Input: part model. Units: mm. Frame: model coordinates. A direction names the side the tool comes from. Coordinates: 2 decimals unless noted, no trailing zeros. Order: outer loops, then holes, each group sorted by start corner. A loop starts at its lowest first (then second) coordinate and runs counter-clockwise, first axis right, second up. Notation, with made-up numbers: (84.25, 65) - (123.25, 65) arc R34 cw to (123.25, 100) - close; hole circle Ø7 at (-0.5, 13). An arc over 180 degrees is marked (long way). Answer as CSV lines item,"result". Start each with the question number.
Item 1: First-contact query: pin 1 (6 mm diameter, centred on y = 2, z = 8.5, fed in from +X); pin 2 (10 mm diameter, centred on x = 57.5, y = 29.5, fed in from -Z); pin 3 (10 mm diameter, centred on x = 17, z = 5, fed in from -Y). Flat tips, straight axial feed; report the tip coordinate or a pass-through.
Item 2: Section C-C (x = 61). Output: boundary loops of the cut face in (y, z), and give its area (3 significant figures).
Item 3: Section D-D (z = 2.5). Output: boundary loops of the cut face in (x, y), and give its area (3 significant figures).
Item 4: Access query for faces 1 (the flat face through (45, 25, 5)), 2 (the flat face through (45, 25, 15)), 3 (the flat face through (45, 15, 10)), 4 (the flat face through (0, 0, 0)). Directions: +Z, -Z, +X, -X, +Y, -Y. A direction counts if a zero-diameter tool reaches every point of the face in a straight line with its end or side. Return the directions, or none.
Item 5: Section A-A (y = 26). Output: boundary loops of the cut face in (x, z), and give its area (3 significant figures).
Item 6: Section B-B (z = 9.5). Output: boundary loops of the cut face in (x, y), and give its area (3 significant figures).
Item 7: Material intervals for line 1 along X through (y, z) = (12.5, 1.5); line 2 along Z through (x, y) = (56, 17.5); line 3 along Y through (x, z) = (18, 8.75), sorted ascending.
from build123d import *

# Parameters (mm, degrees)
F0_W     = 20
F0_H     = 70
F1_DEPTH = 20
F2_W     = 20
F2_H     = 10
F3_DEPTH = 70


with BuildPart() as f1:
    # F0 (on Top) → F1 (new body)
    with BuildSketch(Plane.XY):
        Rectangle(F0_W, F0_H)
    extrude(amount=F1_DEPTH)

    # F2 (on face) → F3 (join)
    with BuildSketch(Plane.YZ.offset(10)):
        with Locations((25, 10)):
            Rectangle(F2_W, F2_H)
    extrude(amount=F3_DEPTH)


solid = f1.part
Determined:
1,pin 1,"stops at x = 10"
1,pin 2,"stops at z = 5"
1,pin 3,"stops at y = 15"
2,outline,"(15, 5) - (35, 5) - (35, 15) - (15, 15) - close"
2,area,"200 mm^2"
3,outline,"(-10, -35) - (10, -35) - (10, 35) - (-10, 35) - close"
3,area,"1,400 mm^2"
4,face 1,"-Z, +X, +Y, -Y"
4,face 2,"+Z, +X, +Y, -Y"
4,face 3,"+Z, -Z, +X, -Y"
4,face 4,"-Z, +X, -X, +Y, -Y"
5,outline,"(-10, 0) - (10, 0) - (10, 5) - (80, 5) - (80, 15) - (10, 15) - (10, 20) - (-10, 20) - close"
5,area,"1,100 mm^2"
6,outline,"(-10, -35) - (10, -35) - (10, 15) - (80, 15) - (80, 35) - (-10, 35) - close"
6,area,"2,800 mm^2"
7,line 1,"x = -10 to 10"
7,line 2,"z = 5 to 15"
7,line 3,"y = 15 to 35"
